Work out the finished part from the listing and answer in its coordinate system (mm). Coordinates: 2 decimals unless noted, no trailing zeros. Loops run counter-clockwise (first coordinate to the right, second up) from the corner with the lowest first, then second, coordinate; pieces in that order, holes last. Notation, with made-up numbers: (-34, 5) - (-26, 5) arc R16 cw to (-26, 35) - close; hole circle Ø10 at (78.5, 56.5). An arc over 180 degrees is marked (long way). Write each question's results on one line, items separated by ' | '. Start each with the question number.
1. A cutting plane is placed at A-A on z = 60. Determine the outline of the cut face in (x, y).
2. A cutting plane is placed at C-C on y = 1.45. Determine the outline of the cut face in (x, z).
3. Find the intervals of material crossed by line 1 along Z through (x, y) = (-34.5, 0.3); line 2 along Z through (x, y) = (-4.5, 1.4); line 3 along Z through (x, y) = (-14.5, 0.6), in increasing order. Write a range as [from, to].
4. This flat-tipped pin is pushed along its axis until it touches: P1, Ø1, axis at y = 1, z = 85.5, coming from the -X side. Where does it stop, or does it pass through?
5. A cutting plane is placed at B-B on x = -59.5. Determine the outline of the cut face in (y, z), then the cut area to 3 significant figures.
from build123d import *

# Parameters (mm, degrees)
BOSS_EXTRUDE1_DEPTH = 3


with BuildPart() as part:
    # Sketch2 → Boss-Extrude1 (new body)
    with BuildSketch(Plane(origin=(0, 0, 0), x_dir=(-1, 0, 0), z_dir=(0, 1, 0))):
        with BuildLine():
            Line((0, 0), (70, 0))
            ThreePointArc((70, 0), (87.015622115, 29.654658201), (98.389955297, 61.896784273))
            ThreePointArc((98.389955297, 61.896784273), (97.649210784, 74.044604409), (90.003901507, 83.513895964))
            ThreePointArc((90.003901507, 83.513895964), (47.456729901, 99.2211161), (2.347235642, 94.518765226))
            ThreePointArc((2.347235642, 94.518765226), (-0.943195566, 90.666547418), (0.820695537, 85.917315086))
            ThreePointArc((0.820695537, 85.917315086), (21.067224953, 42.761339844), (0, 0))
        make_face()
    extrude(amount=BOSS_EXTRUDE1_DEPTH)


solid = part.part
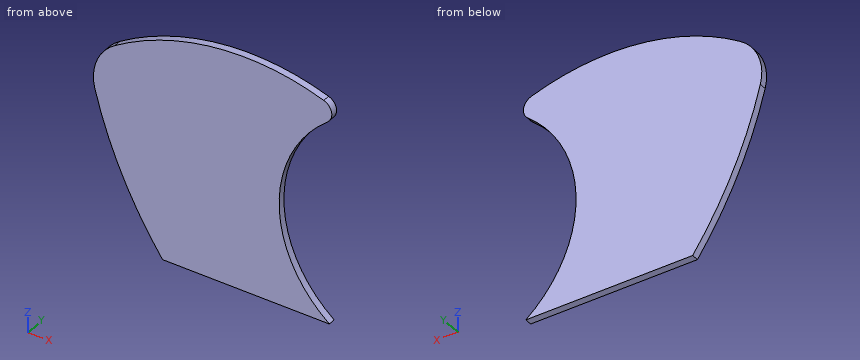
Values:
1) outline: (-97.9, 0) - (-18.47, 0) - (-18.47, 3) - (-97.9, 3) - close
2) outline: (-98.39, 61.9) arc R188.34 ccw to (-70, 0) - (0, 0) arc R55 cw to (-0.82, 85.92) arc R5 ccw to (-2.35, 94.52) arc R100 ccw to (-90, 83.51) arc R20 ccw to start
3) line 1: [0, 100] | line 2: [0, 3.94], [82.63, 95.24] | line 3: [0, 17.22], [69.35, 97.88]
4) P1: x = -87.68
5) outline: (0, 0) - (3, 0) - (3, 96.95) - (0, 96.95) - close | area: 291 mm^2
